The model under review builds one solid part; all positions refer to its coordinate system, in mm. A direction names the side the tool comes from. Coordinates: 2 decimals unless noted, no trailing zeros. Order: outer loops, then holes, each group sorted by start corner. A loop starts at its lowest first (then second) coordinate and runs counter-clockwise, first axis right, second up. Notation, with made-up numbers: (21, 21) -> (66, 21) arc R13 ccw to (66, 43) -> close; hole circle Ø10 at (10.5, 54.5). An arc over 180 degrees is marked (long way). Use one line per item in the form item = value. Start each with the question number.
(1) For faces 1 (the flat face through (-3.5, 49.4, 3)), 2 (the cylindrical face through (0.219, 49.346, 2.165)), 3 (the cylindrical face through (-1.125, 10.54, 1.007)), list the 3-axis set-ups (+Z, -Z, +X, -X, +Y, -Y) from which the entire face can be reached by the end or side of a thin tool; tool diameter is ignored.
(2) Wall thickness on line 1 along Z through (x, y) = (-5, 24); line 2 along X through (y, z) = (31, 1.25); line 3 along Y through (x, z) = (-5, 1.6): over which ranges is each line inside the solid? List them lowest first.
(3) Take a section at B-B (y = 9). State the section outline as (x, z) points.
(4) Take a section at C-C (y = 42.5). State the section outline as (x, z) points.
(5) Take a section at A-A (z = 2.95). State the section outline as (x, y) points, then the cut area to 3 significant figures.
(6) Insertion check: pin 1 Ø0.6 at (x, y) = (-0.5, 11.5) entering from +Z; pin 2 Ø1.8 at (y, z) = (49, 4) entering from -X; pin 3 Ø0.8 at (x, y) = (-5.5, 49) entering from +Z. Each pin has a flat end and moves straight along its axis. Give the tip position at first contact, or say it passes through.
(7) Mouldability with a two-part tool opening along X and no side actions: class faces 4 (the flat face through (-6.5, 49.4, 3)), 5 (the flat face through (0, 26, 1)), 6 (the flat face through (-5.035, 48.125, 1.688)) as +X half, -X half, draft (parallel to the pull), parting line (faces both ways), or undercut.
```python
from build123d import *

# Parameters (mm, degrees)
F0_W         = 10
F0_H         = 52
F1_DEPTH     = 1.5
F2_W         = 5
F2_H         = 2
F3_DEPTH     = 3
F5_DEPTH     = 6
F7_DEPTH     = 1
F8_DEPTH     = 12
F9_R         = 1.5
F10_R        = 1.5
F12_DEPTH    = 1
F13_T1_DEPTH = 25.612494996
F14_W        = 3
F14_H        = 2.5
F15_DEPTH    = 5


# Not quite as in the source:
# - a fillet or chamfer that OpenCascade refuses, or shapes differently, is made with other operations: its cross-section is extruded or revolved along the edge and cut away or added


with BuildPart() as f1:
    # F0 (on Top) → F1 (new body)
    with BuildSketch(Plane.XY):
        with Locations((-5, 26)):
            Rectangle(F0_W, F0_H)
    extrude(amount=F1_DEPTH)

    # F2 (on face) → F3 (join)
    with BuildSketch(Plane.XY.offset(1.5)):
        with Locations((-5, 49)):
            Rectangle(F2_W, F2_H)
    extrude(amount=F3_DEPTH)

    # F4 (on face) → F5 (cut)
    with BuildSketch(Plane(origin=(-7.5, 0, 0), x_dir=(0, -1, 0), z_dir=(-1, 0, 0))):
        Polygon((-48, 4.5), (-50, 4.5), (-48, 1.5), align=None)
    extrude(amount=-F5_DEPTH, mode=Mode.SUBTRACT)

    # F6 (on face) → F7 (join)
    with BuildSketch(Plane(origin=(-10, 0, 0), x_dir=(0, -1, 0), z_dir=(-1, 0, 0))):
        with BuildLine():
            Line((-49.75, 1.5), (-48.25, 1.5))
            ThreePointArc((-48.25, 1.5), (-49, 2.25), (-49.75, 1.5))
        make_face()
        with BuildLine():
            ThreePointArc((-49.75, 1.5), (-49, 0.75), (-48.25, 1.5))
            Line((-48.25, 1.5), (-49.75, 1.5))
        make_face()
    extrude(amount=F7_DEPTH)

    # F6 (on face) → F8 (join)
    with BuildSketch(Plane(origin=(-10, 0, 0), x_dir=(0, -1, 0), z_dir=(-1, 0, 0))):
        with BuildLine():
            Line((-49.75, 1.5), (-48.25, 1.5))
            ThreePointArc((-48.25, 1.5), (-49, 2.25), (-49.75, 1.5))
        make_face()
        with BuildLine():
            ThreePointArc((-49.75, 1.5), (-49, 0.75), (-48.25, 1.5))
            Line((-48.25, 1.5), (-49.75, 1.5))
        make_face()
    extrude(amount=-F8_DEPTH)

    # F9
    f9_edges = [f1.edges().sort_by_distance(p)[0] for p in [
        (-10, 0, 0.75),
    ]]
    fillet(f9_edges, radius=F9_R)

    # F10
    f10_edges = [f1.edges().sort_by_distance(p)[0] for p in [
        (0, 0, 0.75),
    ]]
    fillet(f10_edges, radius=F10_R)

    # F11 (on face) → F12 (cut)
    with BuildSketch(Plane.XY.offset(1.5)):
        with BuildLine():
            Line((0, 7.928885867), (0, 13.071114133))
            ThreePointArc((0, 13.071114133), (-1.1252637799, 10.5), (0, 7.928885867))
        make_face()
    extrude(amount=-F12_DEPTH, mode=Mode.SUBTRACT)

    # F13: fillet of radius 4 on 1 edges, made by hand

    # F13_s2 → F13_t1 (cut)
    with BuildSketch(Plane.YZ.offset(-17.806247498)):
        with BuildLine():
            ThreePointArc((48.8775010008, 0), (50.6095518084, 0.3944487245), (52, 1.5))
            Line((52, 1.5), (52, 0))
            Line((52, 0), (48.8775010008, 0))
        make_face()
    extrude(amount=F13_T1_DEPTH, mode=Mode.SUBTRACT)

    # F14 (on face) → F15 (cut)
    with BuildSketch(Plane(origin=(0, 50, 0), x_dir=(-1, 0, 0), z_dir=(0, 1, 0))):
        with Locations((5, 3.25)):
            Rectangle(F14_W, F14_H)
    extrude(amount=-F15_DEPTH, mode=Mode.SUBTRACT)


solid = f1.part
```
Findings:
q1.face_1 = +Z, +Y, -Y
q1.face_2 = +X
q1.face_3 = +Z, +X
q2.line_1 = 0 to 1.5
q2.line_2 = -10 to 0
q2.line_3 = 48.07 to 50
q3.outline = (-10, 0) -> (0, 0) -> (0, 0.5) -> (-0.79, 0.5) -> (-0.79, 1.5) -> (-10, 1.5) -> close
q4.outline = (-10, 0) -> (0, 0) -> (0, 1.5) -> (-10, 1.5) -> close
q5.outline = (-7.5, 48.97) -> (-6.5, 48.97) -> (-6.5, 50) -> (-7.5, 50) -> close; (-3.5, 48.97) -> (-2.5, 48.97) -> (-2.5, 50) -> (-3.5, 50) -> close
q5.area = 2.07 mm²
q6.pin_1 = 0.5
q6.pin_2 = -7.5
q6.pin_3 = 2
q7.face_4 = undercut
q7.face_5 = +X half
q7.face_6 = draft
